from build123d import *

# Parameters (mm, degrees)
CROQUIS1_R                 = 8.5
SALIENTE_EXTRUIR1_DEPTH    = 15
CORTAR_EXTRUIR1_DEPTH      = 9
CROQUIS9_R                 = 11.15
SALIENTE_EXTRUIR5_DEPTH    = 10
CROQUIS3_R                 = 9.53
CORTAR_EXTRUIR2_DEPTH      = 9
CORTAR_EXTRUIR4_DEPTH      = 22.763386685
CORTAR_EXTRUIR4_DEPTH_BACK = 22.763386685
CROQUIS5_R                 = 2.025
CROQUIS7_R                 = 8.5
SALIENTE_EXTRUIR3_DEPTH    = 3
CROQUIS10_W                = 5.42
CROQUIS10_H                = 2.48
CORTAR_EXTRUIR5_DEPTH      = 6
CROQUIS12_R                = 1.25
CORTAR_EXTRUIR6_DEPTH      = 24.930002183


with BuildPart() as part:
    # Croquis1 → Saliente-Extruir1 (new body)
    with BuildSketch(Plane(origin=(0, 0, 0), x_dir=(0, 0, -1), z_dir=(1, 0, 0))):
        Circle(CROQUIS1_R)
    extrude(amount=SALIENTE_EXTRUIR1_DEPTH)

    # Croquis2 → Cortar-Extruir1 (cut)
    with BuildSketch(Plane(origin=(15, 0, 0), x_dir=(0, 0, -1), z_dir=(1, 0, 0))):
        with BuildLine():
            Line((-1.457669373, -1.34), (1.457669373, -1.34))
            ThreePointArc((1.457669373, -1.34), (0, 1.98), (-1.457669373, -1.34))
        make_face()
    extrude(amount=-CORTAR_EXTRUIR1_DEPTH, mode=Mode.SUBTRACT)

    # Croquis9 → Saliente-Extruir5 (add)
    with BuildSketch(Plane.ZY):
        Circle(CROQUIS9_R)
    extrude(amount=-SALIENTE_EXTRUIR5_DEPTH)

    # Croquis3 → Cortar-Extruir2 (cut)
    with BuildSketch(Plane.ZY):
        Circle(CROQUIS3_R)
    extrude(amount=-CORTAR_EXTRUIR2_DEPTH, mode=Mode.SUBTRACT)

    # Croquis5 → Cortar-Extruir4 (cut, two sides: drawn at the far end of the back side and taken through both)
    with BuildSketch(Plane.XY.offset(-CORTAR_EXTRUIR4_DEPTH_BACK)):
        with Locations((5, 0)):
            Circle(CROQUIS5_R)
    extrude(amount=CORTAR_EXTRUIR4_DEPTH + CORTAR_EXTRUIR4_DEPTH_BACK, mode=Mode.SUBTRACT)

    # Croquis7 → Saliente-Extruir3 (add)
    with BuildSketch(Plane(origin=(15, 0, 0), x_dir=(0, 0, -1), z_dir=(1, 0, 0))):
        with Locations(Location((0, 0, 0), (0, 0, 180))):
            Circle(CROQUIS7_R)
        with BuildLine():
            Line((-1.457669373, -1.34), (1.457669373, -1.34))
            ThreePointArc((1.457669373, -1.34), (0, 1.98), (-1.457669373, -1.34))
        make_face(mode=Mode.SUBTRACT)
    extrude(amount=SALIENTE_EXTRUIR3_DEPTH)

    # Redondeo1: read off the stored shape, not the designer's step
    # Redondeo1 outline → Redondeo1 (revolve)
    with BuildSketch(Plane.YX):
        with BuildLine():
            Line((8.5, 10), (11.15, 10))
            ThreePointArc((11.15, 10), (9.186031995, 13.140616114), (8.5, 16.780671058))
            Line((8.5, 16.780671058), (8.5, 10))
        make_face()
    revolve(axis=Axis((0, 0, 0), (1, 0, 0)))

    # Croquis10 → Cortar-Extruir5 (cut)
    with BuildSketch(Plane(origin=(18, 0, 0), x_dir=(0, 0, -1), z_dir=(1, 0, 0))):
        with Locations((0, -4.18)):
            Rectangle(CROQUIS10_W, CROQUIS10_H)
    extrude(amount=-CORTAR_EXTRUIR5_DEPTH, mode=Mode.SUBTRACT)

    # Croquis12 → Cortar-Extruir6 (cut, through all)
    with BuildSketch(Plane(origin=(0, 0, 0), x_dir=(1, 0, 0), z_dir=(0, 1, 0))):
        with Locations(Location((14.65, 0, 0), (0, 0, 140.139668223))):
            Circle(CROQUIS12_R)
    extrude(amount=-CORTAR_EXTRUIR6_DEPTH, mode=Mode.SUBTRACT)


solid = part.part
Could you check a few things on this model? Use its own coordinates, in mm. A direction names the side the tool comes from. Coordinates: 2 decimals unless noted, no trailing zeros. Order: outer loops, then holes, each group sorted by start corner. A loop starts at its lowest first (then second) coordinate and runs counter-clockwise, first axis right, second up. Notation, with made-up numbers: (87.5, -2.75) - (137.5, -2.75) arc R13 cw to (137.5, 16.25) - close; hole circle Ø3 at (-7, 7.5). An arc over 180 degrees is marked (long way). Answer in a Markdown table with one row per item. Add a question column.
(1) On a 3-axis mill with a long thin cutter (end or side, diameter ignored), from which of +Z, -Z, +X, -X, +Y, -Y can I reach the whole of each face in a straight line? I mean faces 1 (the face through (17.38, -2.55, 8.11)), 2 (the face through (18, 2, 2)), 3 (the face through (4.44, 2.86, 9.09)), 4 (the face through (2.977, 0.089, -10.244)), 5 (the face through (13.46, -7.23, 0.38)). Say none if no direction works.
(2) If we section it at A-A, the plane y = 0: Please give me the cut outline in (x, z) (3 decimals).
(3) If we section it at C-C, the plane x = 5: Please give me the cut outline in (y, z) (3 decimals), then the cut area to 3 significant figures.
(4) Will these pins go through, and if not, where does the flat tip stop? pin 1 (2.5 mm diameter, centred on x = 14.5, z = 0, fed in from -Y); pin 2 (1.5 mm diameter, centred on x = 14.5, z = 0.5, fed in from +Y); pin 3 (5.5 mm diameter, centred on y = 2, z = -4.5, fed in from -X); pin 4 (5.5 mm diameter, centred on x = 5, y = 0, fed in from +Z).
(5) If we section it at B-B, the plane z = 0: Please give me the cut outline in (x, y), then the cut area to 3 significant figures.
(6) I need wall thicknesses on L1, parallel to X at y = -6.6, z = 0; L2, parallel to Y at x = 3.25, z = 0; L3, parallel to Y at x = 4.75, z = -5.75. Which ranges of each line are inside material? Lowest first, please.
(7) If we section it at D-D, the plane x = 14.65: Please give me the cut outline in (y, z), then the cut area to 3 significant figures.
(8) If we mould it in two halves opening along Z, with no side actions, what happens to faces 6 (the face through (13, -1.34, 0)), 7 (the face through (0, 8.3, -5)), 8 (the face through (4.93, 3.349, 10.635))? For each: released by +Z, released by -Z, zero draft, split by the parting line, or undercut.
Results are:
| question | item | result |
|---|---|---|
| 1 | face 1 | +X |
| 1 | face 2 | +Z, -Z, +X, +Y, -Y |
| 1 | face 3 | -X |
| 1 | face 4 | +Z, -Z |
| 1 | face 5 | -Y |
| 2 | outline | (0, -11.15) - (2.975, -11.15) - (2.975, -9.53) - (0, -9.53) - close; (0, 9.53) - (2.975, 9.53) - (2.975, 11.15) - (0, 11.15) - close; (7.025, -11.15) - (10, -11.15) arc R10 cw to (16.781, -8.5) - (18, -8.5) - (18, -1.98) - (10, -1.98) - (10, 1.98) - (18, 1.98) - (18, 8.5) - (16.781, 8.5) arc R10 cw to (10, 11.15) - (7.025, 11.15) - (7.025, 9.53) - (9, 9.53) - (9, -9.53) - (7.025, -9.53) - close |
| 3 | outline | (-2.025, -10.965) - (-2.025, -9.312) arc R9.53 cw to (-2.025, 9.312) - (-2.025, 10.965) arc R11.15 ccw to start; (2.025, -10.965) arc R11.15 ccw to (2.025, 10.965) - (2.025, 9.312) arc R9.53 cw to (2.025, -9.312) - close |
| 3 | area | 92.0 mm2 |
| 4 | pin 1 | stops at y = -9.14 |
| 4 | pin 2 | stops at y = 8.96 |
| 4 | pin 3 | stops at x = 9 |
| 4 | pin 4 | stops at z = 11.15 |
| 5 | outline | (0, -11.15) - (10, -11.15) arc R10 cw to (13.4, -9.09) - (13.4, -5.42) - (12, -5.42) - (12, -2.94) - (13.4, -2.94) - (13.4, -1.34) - (10, -1.34) - (10, 1.98) - (18, 1.98) - (18, 8.5) - (16.78, 8.5) arc R10 cw to (10, 11.15) - (0, 11.15) - (0, 9.53) - (9, 9.53) - (9, -9.53) - (0, -9.53) - close; (15.9, -8.54) arc R10 cw to (16.78, -8.5) - (18, -8.5) - (18, -5.42) - (15.9, -5.42) - close; (15.9, -2.94) - (18, -2.94) - (18, -1.34) - (15.9, -1.34) - close |
| 5 | area | 145 mm2 |
| 6 | L1 | x = 9 to 13.4, 15.9 to 18 |
| 6 | L2 | y = -11.15 to -9.53, 9.53 to 11.15 |
| 6 | L3 | y = -9.55 to -7.6, 7.6 to 9.55 |
| 7 | outline | (-8.64, -1.25) arc R8.73 ccw (long way) to (-8.64, 1.25) - (-5.42, 1.25) - (-5.42, 2.71) - (-2.94, 2.71) - (-2.94, 1.25) - (-1.34, 1.25) - (-1.34, 1.46) arc R1.98 cw (long way) to (-1.34, -1.46) - (-1.34, -1.25) - (-2.94, -1.25) - (-2.94, -2.71) - (-5.42, -2.71) - (-5.42, -1.25) - close |
| 7 | area | 203 mm2 |
| 8 | face 6 | undercut |
| 8 | face 7 | zero draft |
| 8 | face 8 | split by the parting line |
